```python
from build123d import *

# Parameters (mm, degrees)
SKETCH2_W                 = 25.4
SKETCH2_H                 = 3
BOSS_EXTRUDE1_DEPTH       = 70
SKETCH4_R                 = 30
BOSS_EXTRUDE2_DEPTH       = 10
SKETCH5_R                 = 30
SKETCH5_R_2               = 20
BOSS_EXTRUDE3_DEPTH       = 70
SKETCH8_R                 = 24.75
SKETCH8_R_2               = 20
BOSS_EXTRUDE4_DEPTH       = 20
SKETCH9_R                 = 1.5
CUT_EXTRUDE4_DEPTH        = 29.5
CUT_EXTRUDE4_DEPTH_BACK   = 32.5
F_4_40_TAPPED_HOLE1_D     = 2.2606
F_4_40_TAPPED_HOLE1_DEPTH = 7.6
F_4_40_TAPPED_HOLE1_TIP   = 0.679152758
SKETCH3_R                 = 3
CUT_EXTRUDE5_DEPTH        = 10


with BuildPart() as part:
    # Sketch2 → Boss-Extrude1 (new body)
    with BuildSketch(Plane(origin=(0, 0, 0), x_dir=(1, 0, 0), z_dir=(0, 1, 0))):
        with Locations((12.7, 1.5)):
            Rectangle(SKETCH2_W, SKETCH2_H)
    extrude(amount=BOSS_EXTRUDE1_DEPTH)

    # Sketch4 → Boss-Extrude2 (add)
    with BuildSketch(Plane(origin=(0, 70, 0), x_dir=(1, 0, 0), z_dir=(0, 1, 0))):
        with Locations((12.7, 1.5)):
            Circle(SKETCH4_R)
    extrude(amount=BOSS_EXTRUDE2_DEPTH)

    # Sketch5 → Boss-Extrude3 (add)
    with BuildSketch(Plane(origin=(0, 80, 0), x_dir=(1, 0, 0), z_dir=(0, 1, 0))):
        with Locations((12.7, 1.5)):
            Circle(SKETCH5_R)
        with Locations((12.7, 1.5)):
            Circle(SKETCH5_R_2, mode=Mode.SUBTRACT)
    extrude(amount=BOSS_EXTRUDE3_DEPTH)

    # Sketch8 → Boss-Extrude4 (add)
    with BuildSketch(Plane(origin=(0, 150, 0), x_dir=(1, 0, 0), z_dir=(0, 1, 0))):
        with Locations((12.7, 1.5)):
            Circle(SKETCH8_R)
        with Locations((12.7, 1.5)):
            Circle(SKETCH8_R_2, mode=Mode.SUBTRACT)
    extrude(amount=BOSS_EXTRUDE4_DEPTH)

    # Sketch9 → Cut-Extrude4 (cut, two sides)
    with BuildSketch(Plane.XY) as cut_extrude4_sk:
        with Locations((12.7, 160)):
            Circle(SKETCH9_R)
    extrude(amount=CUT_EXTRUDE4_DEPTH, mode=Mode.SUBTRACT)
    extrude(cut_extrude4_sk.sketch, amount=-CUT_EXTRUDE4_DEPTH_BACK, mode=Mode.SUBTRACT)

    # #4-40 Tapped Hole1
    with Locations(Plane.XY):
        with Locations((12.7, 22.2), (20.927241336, 17.45), (20.927241336, 7.95), (12.7, 3.2), (4.472758664, 7.95), (4.472758664, 17.45)):
            Hole(F_4_40_TAPPED_HOLE1_D / 2, depth=F_4_40_TAPPED_HOLE1_DEPTH)
            with Locations((0, 0, -(F_4_40_TAPPED_HOLE1_DEPTH + F_4_40_TAPPED_HOLE1_TIP / 2))):  # 118° drill point
                Cone(0, F_4_40_TAPPED_HOLE1_D / 2, F_4_40_TAPPED_HOLE1_TIP, mode=Mode.SUBTRACT)

    # Sketch3 → Cut-Extrude5 (cut)
    with BuildSketch(Plane.XY):
        with Locations((12.7, 12.7)):
            Circle(SKETCH3_R)
    extrude(amount=-CUT_EXTRUDE5_DEPTH, mode=Mode.SUBTRACT)


solid = part.part
```
Could you check a few things on this model? Use its own coordinates, in mm. A direction names the side the tool comes from. Coordinates: 2 decimals unless noted, no trailing zeros. Write each loop counter-clockwise with the first axis right and the second up, starting at its lowest first coordinate (ties: lowest second). Pieces come first, ordered by that corner, then holes. Notation, with made-up numbers: M -38,51 L 1,51 A13 ccw 1,61 Z; hole C -32,-20 d5. An arc over 180 degrees is marked long. Answer as CSV lines item,"result". Start each with the question number.
1) For P1, Ø4, axis at x = 17.5, y = 124, coming from the -Z side; P2, Ø3, axis at x = 11.5, z = 7, coming from the -Y side; P3, Ø20.5, axis at x = 15.5, y = 45, coming from the +Z side, each with a flat end and sliding along its axis, tell me the tip position at first contact or that it passes through.
2) Please list where these lines run through material, in increasing order: line 1 (Y direction, x = 12.7, z = -1.05); line 2 (X direction, y = 3, z = -1); line 3 (X direction, y = 148, z = -1). Write a range as from..to.
3) We'd pull the mould along X, two halves only. Please class faces 6 (the flat face through (25.4, 35, -1)), 7 (the flat face through (13, 0, -2)), 8 (the cylindrical face through (14.31, 15.23, -1.48)), 9 (the cylindrical face through (12.505, 161.487, -23.813)): +X half, -X half, draft (parallel to the pull), parting line (faces both ways), or undercut.
4) For faces 1 (the flat face through (13, 35, 0)), 2 (the flat face through (13, 35, -3)), 3 (the flat face through (0, 35, -1)), 4 (the flat face through (12, 80, -2)), 5 (the flat face through (33, 170, -2)), which set-ups out of +Z, -Z, +X, -X, +Y, -Y let a thin tool reach every point of the face, with its end or its side?
5) I want a section at C-C, the plane y = 154. Please give me the cut outline in (x, z), and give its area (3 significant figures).
6) I want a section at A-A, the plane y = 97. Please give me the cut outline in (x, z), and give its area (3 significant figures).
7) I want a section at B-B, the plane z = -8.5. Please give me the cut outline in (x, y) (3 decimals), and give its area (3 significant figures).
Data:
1,P1,"stops at z = -31.37"
1,P2,"stops at y = 70"
1,P3,"stops at z = 0"
2,line 1,"y = 0..2.07, 4.33..9.7, 15.7..21.07, 23.33..80"
2,line 2,"x = 0..11.59, 13.81..25.4"
2,line 3,"x = -17.3..-7.29, 32.69..42.7"
3,face 6,"+X half"
3,face 7,"draft"
3,face 8,"undercut"
3,face 9,"undercut"
4,face 1,"+Z, +X, -X, -Y"
4,face 2,"-Z, +X, -X, -Y"
4,face 3,"+Z, -Z, -X, -Y"
4,face 4,"+Y"
4,face 5,"+Z, -Z, +X, -X, +Y"
5,outline,"C 12.7,-1.5 d49.5; hole C 12.7,-1.5 d40"
5,area,"668 mm^2"
6,outline,"C 12.7,-1.5 d60; hole C 12.7,-1.5 d40"
6,area,"1,570 mm^2"
7,outline,"M -16.472,70 L 41.872,70 L 41.872,150 L 36.439,150 L 36.439,170 L 31.435,170 L 31.435,80 L -6.035,80 L -6.035,170 L -11.039,170 L -11.039,150 L -16.472,150 Z"
7,area,"2,240 mm^2"
